The drawing under review shows one solid part. Ordinate dimensions are in mm from its lowest x, y, z. A direction names the side the tool comes from. Coordinates: 2 decimals unless noted, no trailing zeros. Loops run counter-clockwise (first coordinate to the right, second up) from the corner with the lowest first, then second, coordinate; pieces in that order, holes last. Notation, with made-up numbers: M -11.5,66.25 L 1.5,66.25 A20 cw 1.5,100.25 Z; hole C -15,16 d4. An arc over 180 degrees is marked long. Answer as a JSON object with one key per item and string values. Group by question number.
1. Consider section C-C (z = 7.75). State the section outline as (x, y) points, then the cut area to 3 significant figures.
2. Consider section B-B (y = 18.5). State the section outline as (x, z) points, then the cut area to 3 significant figures.
3. To check wall thickness, follow probe 1 along X at (y, z) = (18.5, 0.65); probe 2 along Y at (x, z) = (42.5, 1.25); probe 3 along Z at (x, y) = (25, 3.25). State the ranges of each line that lie inside material, in increasing order.
4. Consider section A-A (x = 1.5). State the section outline as (y, z) points.
5. Consider section D-D (x = 10.5). State the section outline as (y, z) points, then the cut area to 3 significant figures.
6. Insertion check: pin 1 (1 mm diameter, centred on x = 36.5, z = 5, fed in from +Y); pin 2 (3 mm diameter, centred on x = 42.5, y = 1.5, fed in from +Z); pin 3 (1.5 mm diameter, centred on y = 11.5, z = 9, fed in from +X). Each pin has a flat end and moves straight along its axis. Give the tip position at first contact, or say it passes through.
7. Machinability: for the marked faces 1 and 2, which of the approach directions +Z, -Z, +X, -X, +Y, -Y give a long, thin tool a straight path to every point of the face, cutting with its end or side? Answer none if there is none.
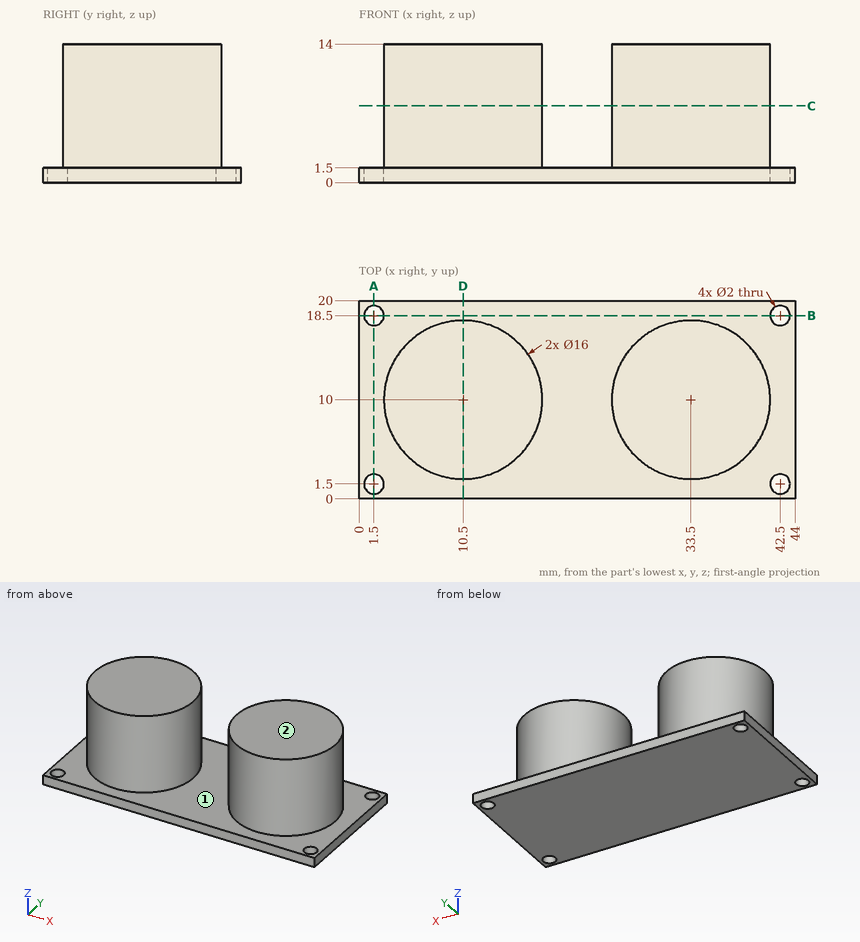
Findings below:
{
 "1": {"outline": "C 10.5,10 d16; C 33.5,10 d16", "area": "402 mm^2"},
 "2": {"outline": "M 0,0 L 0.5,0 L 0.5,1.5 L 0,1.5 Z; M 2.5,0 L 41.5,0 L 41.5,1.5 L 2.5,1.5 Z; M 43.5,0 L 44,0 L 44,1.5 L 43.5,1.5 Z", "area": "60.0 mm^2"},
 "3": {"probe 1": "x = 0 to 0.5, 2.5 to 41.5, 43.5 to 44", "probe 2": "y = 0 to 0.5, 2.5 to 17.5, 19.5 to 20", "probe 3": "z = 0 to 1.5"},
 "4": {"outline": "M 0,0 L 0.5,0 L 0.5,1.5 L 0,1.5 Z; M 2.5,0 L 17.5,0 L 17.5,1.5 L 2.5,1.5 Z; M 19.5,0 L 20,0 L 20,1.5 L 19.5,1.5 Z"},
 "5": {"outline": "M 0,0 L 20,0 L 20,1.5 L 18,1.5 L 18,14 L 2,14 L 2,1.5 L 0,1.5 Z", "area": "230 mm^2"},
 "6": {"pin 1": "stops at y = 17.6", "pin 2": "stops at z = 1.5", "pin 3": "stops at x = 41.46"},
 "7": {"face 1": "+Z", "face 2": "+Z, +X, -X, +Y, -Y"}
}
